Answer from the drawing. Dimensions are ordinates in mm from the lowest x, y and z of the part. A direction names the side the tool comes from. Coordinates: 2 decimals unless noted, no trailing zeros. Write each loop counter-clockwise with the first axis right and the second up, starting at its lowest first coordinate (ties: lowest second). Pieces come first, ordered by that corner, then holes.
(1) Find the intervals of material crossed by probe 1 along Y at (x, z) = (48.5, 5); probe 2 along X at (y, z) = (25.5, 31); probe 3 along X at (y, z) = (37, 23.5), in increasing order.
(2) Section B-B on x = 65 is taken. Write down the section's boundary in (y, z), then the cut area to 3 significant figures.
(3) Which of the six approach directions +Z, -Z, +X, -X, +Y, -Y give full straight-line access (tool end or side, diameter ignored) to the marked faces 1, 2, 3, 4 and 5?
(4) Section C-C on z = 28.5 is taken. Write down the section's boundary in (x, y), then the cut area to 3 significant figures.
(5) Section A-A on z = 34 is taken. Write down the section's boundary in (x, y).
(6) Given pin 1 (6 mm diameter, centred on x = 8.5, z = 33.5, fed in from +Y); pin 2 (2 mm diameter, centred on y = 19, z = 28.5, fed in from -X); pin 3 (12 mm diameter, centred on x = 65, y = 45.5, fed in from +Z); pin 4 (12 mm diameter, centred on y = 49, z = 21, fed in from -X), each flat-ended and moving along its own axis, determine where each tip first touches the part or whether it passes through.
(7) Section D-D on x = 31 is taken. Write down the section's boundary in (y, z).
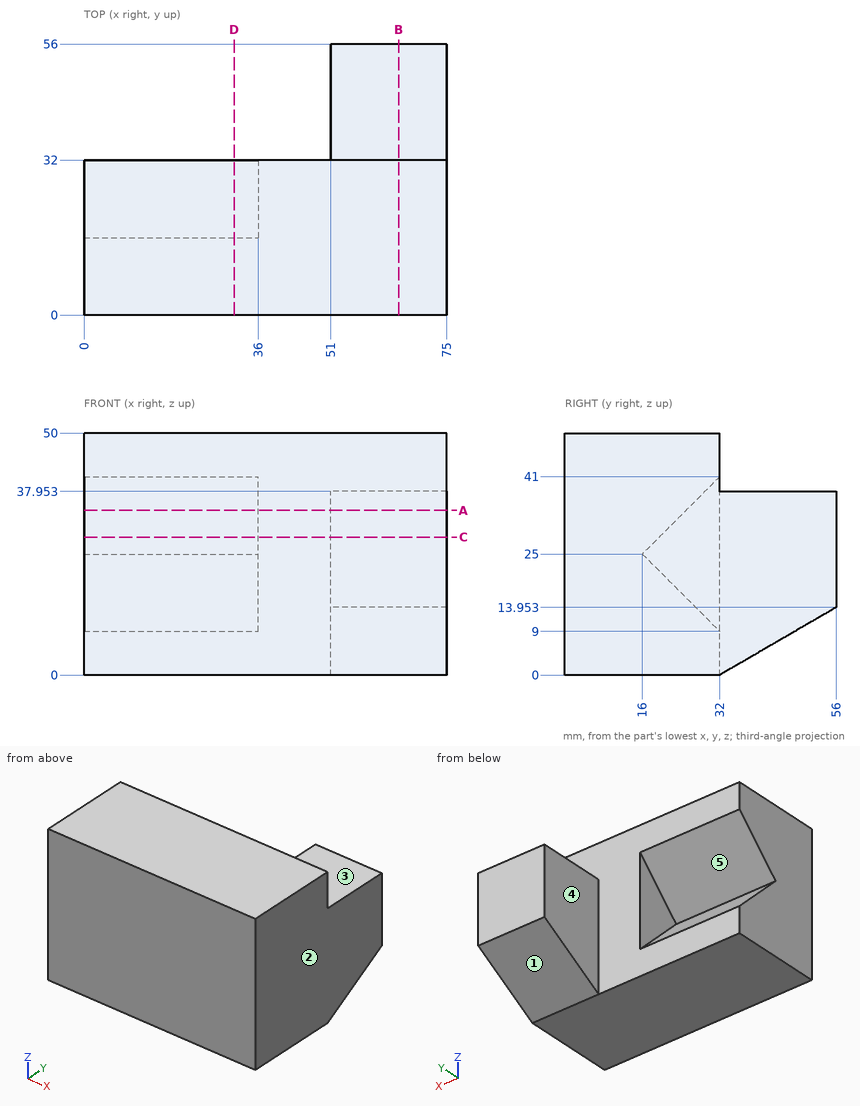
Response:
1. probe 1: y = 0 to 32
1. probe 2: x = 36 to 75
1. probe 3: x = 51 to 75
2. outline: (0, 0) - (32, 0) - (56, 13.95) - (56, 37.95) - (32, 37.95) - (32, 50) - (0, 50) - close
2. area: 2,340 mm2
3. face 1: -Z, +X, -X, +Y
3. face 2: +Z, -Z, +X, +Y, -Y
3. face 3: +Z, +X, -X, +Y
3. face 4: +Z, -Z, -X, +Y
3. face 5: -X, +Y
4. outline: (0, 0) - (75, 0) - (75, 56) - (51, 56) - (51, 32) - (36, 32) - (36, 19.5) - (0, 19.5) - close
4. area: 2,530 mm2
5. outline: (0, 0) - (75, 0) - (75, 56) - (51, 56) - (51, 32) - (36, 32) - (36, 25) - (0, 25) - close
6. pin 1: stops at y = 27.5
6. pin 2: stops at x = 0
6. pin 3: stops at z = 37.95
6. pin 4: stops at x = 51
7. outline: (0, 0) - (32, 0) - (32, 9) - (16, 25) - (32, 41) - (32, 50) - (0, 50) - close
